```python
from build123d import *

# Parameters (mm, degrees)
F1_DEPTH = 5
F2_T     = -1.5
F3_W     = 8.5
F3_H     = 10
F3_W_2   = 1.5
F4_DEPTH = 8.6
F5_W     = 3.2
F5_H     = 4.6355582315
F6_DEPTH = 6
F7_W     = 3.2
F7_H     = 4.6664974656
F8_DEPTH = 6


with BuildPart() as f1:
    # F0 (on Top) → F1 (new body)
    with BuildSketch(Plane.XY):
        Polygon((-0.1638537049, 29.7847446054), (-27.6638537049, 29.7847446054), (-27.6638537049, 19.0347446054), (-27.6638537049, 8.2847446054), (-0.1638537049, 8.2847446054), align=None)
    extrude(amount=F1_DEPTH)

    # F2
    f2_openings = [f1.faces().sort_by_distance(p)[0] for p in [
        (-13.913854, 19.034745, 5),
    ]]
    offset(amount=F2_T, openings=f2_openings)

    # F3 (on face) → F4 (join)
    with BuildSketch(Plane.XY.offset(1.5)):
        with Locations((-5.9138537049, 19.0347446054)):
            Rectangle(F3_W, F3_H)
        with Locations((-0.9138537049, 19.0347446054)):
            Rectangle(F3_W_2, F3_H)
    extrude(amount=-F4_DEPTH)

    # F5 (on face) → F6 (join)
    with BuildSketch(Plane.XZ.offset(-8.2847446054)):
        with Locations((-26.0638537049, 2.3177791158)):
            Rectangle(F5_W, F5_H)
    extrude(amount=F6_DEPTH)

    # F7 (on face) → F8 (join)
    with BuildSketch(Plane(origin=(0, 29.7847446054, 0), x_dir=(-1, 0, 0), z_dir=(0, 1, 0))):
        with Locations((26.0638537049, 2.3332487328)):
            Rectangle(F7_W, F7_H)
    extrude(amount=F8_DEPTH)


solid = f1.part
```
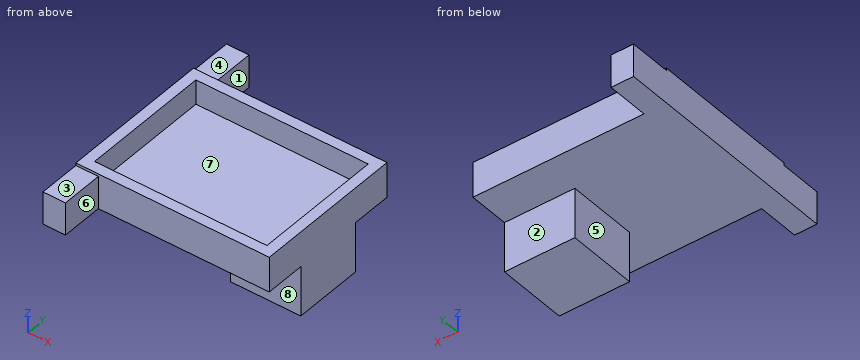
Check sheet for the modelled part. Datum: model origin and axes. Units: mm. Face numbers are marked on the shaded views. A direction names the side the tool comes from. Round coordinates to 2 decimals unless told otherwise and drop trailing zeros. Order: outer loops, then holes, each group sorted by start corner. A loop starts at its lowest first (then second) coordinate and runs counter-clockwise, first axis right, second up. Notation, with made-up numbers: (86.25, 84) -> (112.25, 84) arc R24 ccw to (112.25, 111) -> close; hole circle Ø2 at (-13.75, 78). An arc over 180 degrees is marked (long way). Use CSV: the item, a comma, the result in double quotes.
(1) Depth check by flat-ended pin: pin 1 (3.5 mm diameter, centred on x = -7, z = -4.5, fed in from +Y); pin 2 (1.8 mm diameter, centred on x = -11.5, z = 3, fed in from -Y); pin 3 (3 mm diameter, centred on y = 7.5, z = -3, fed in from +X); pin 4 (2.5 mm diameter, centred on x = -25.5, y = 4.5, fed in from +Z). Enter the tip coordinate at first touch or a pass-through.
Worked out:
pin 1,"y = 24.03"
pin 2,"y = 8.28"
pin 3,"through"
pin 4,"z = 4.64"
(2) Tool access check on the marked faces 1, 2, 3, 4 and 5. Record the directions out of +Z, -Z, +X, -X, +Y, -Y that give a thin tool (end or side, any length) a straight path to the whole face; none if there is none.
Worked out:
face 1,"+Z, -Z, +X, +Y"
face 2,"-Z, +X, -X, +Y"
face 3,"+Z, +X, -X, -Y"
face 4,"+Z, +X, -X, +Y"
face 5,"-Z, -X, +Y, -Y"
(3) Cross-section at A-A (z = 2). Record the boundary of the cut face in (x, y), and give its area (3 significant figures).
Worked out:
outline,"(-27.66, 2.28) -> (-24.46, 2.28) -> (-24.46, 8.28) -> (-0.16, 8.28) -> (-0.16, 29.78) -> (-24.46, 29.78) -> (-24.46, 35.78) -> (-27.66, 35.78) -> close; hole (-26.16, 9.78) -> (-1.66, 9.78) -> (-1.66, 28.28) -> (-26.16, 28.28) -> close"
area,"176 mm²"
(4) Cross-section at D-D (z = -2.5). Record the boundary of the cut face in (x, y), and give its area (3 significant figures).
Worked out:
outline,"(-10.16, 14.03) -> (-0.16, 14.03) -> (-0.16, 24.03) -> (-10.16, 24.03) -> close"
area,"100 mm²"
(5) Cross-section at C-C (x = -9.25). Record the boundary of the cut face in (y, z).
Worked out:
outline,"(8.28, 0) -> (14.03, 0) -> (14.03, -7.1) -> (24.03, -7.1) -> (24.03, 0) -> (29.78, 0) -> (29.78, 5) -> (28.28, 5) -> (28.28, 1.5) -> (9.78, 1.5) -> (9.78, 5) -> (8.28, 5) -> close"
(6) Material ranges on line 1 along Y through (x, z) = (-14.25, 4.75); line 2 along X through (y, z) = (10, 4.75); line 3 along X through (y, z) = (7, 1.25), recorded low to high. Write a range as from..to.
Worked out:
line 1,"8.28..9.78, 28.28..29.78"
line 2,"-27.66..-26.16, -1.66..-0.16"
line 3,"-27.66..-24.46"
(7) Cross-section at B-B (y = 25). Record the boundary of the cut face in (x, z).
Worked out:
outline,"(-27.66, 0) -> (-0.16, 0) -> (-0.16, 5) -> (-1.66, 5) -> (-1.66, 1.5) -> (-26.16, 1.5) -> (-26.16, 5) -> (-27.66, 5) -> close"
(8) Draft check along Y on the marked faces 6, 7 and 8. Enter one of: pulls with the +Y half, pulls with the -Y half, needs draft (parallel to the pull), parting line crosses it, or undercut.
Worked out:
face 6,"needs draft"
face 7,"undercut"
face 8,"pulls with the -Y half"
